```python
from build123d import *

# Parameters (mm, degrees)
F0_W     = 17.78
F0_H     = 12.7
F0_R     = 1.27
F1_DEPTH = 2.54
F2_W     = 2.54
F2_H     = 12.7
F3_DEPTH = 15.24
F4_R     = 1.27
F5_DEPTH = 25.4
F6_SIZE  = 1.27


with BuildPart() as f1:
    # F0 (on Top) → F1 (new body)
    with BuildSketch(Plane.XY):
        with Locations((-26.076857, 25.594209)):
            Rectangle(F0_W, F0_H)
        with Locations((-28.616857, 25.594209)):
            Circle(F0_R, mode=Mode.SUBTRACT)
        with Locations((-20.996857, 25.594209)):
            Circle(F0_R, mode=Mode.SUBTRACT)
    extrude(amount=F1_DEPTH)

    # F2 (on face) → F3 (join)
    with BuildSketch(Plane.XY.offset(2.54)):
        with Locations((-33.696857, 25.594209)):
            Rectangle(F2_W, F2_H)
    extrude(amount=F3_DEPTH)

    # F4 (on face) → F5 (cut)
    with BuildSketch(Plane(origin=(-34.966857, 0, 0), x_dir=(0, -1, 0), z_dir=(-1, 0, 0))):
        with Locations((-25.594209, 13.97)):
            Circle(F4_R)
        with Locations((-25.594209, 6.35)):
            Circle(F4_R)
    extrude(amount=-F5_DEPTH, mode=Mode.SUBTRACT)

    # F6
    f6_edges = [f1.edges().sort_by_distance(p)[0] for p in [
        (-33.696857, 19.244209, 17.78),
        (-33.696857, 31.944209, 17.78),
        (-17.186857, 19.244209, 1.27),
        (-17.186857, 31.944209, 1.27),
    ]]
    chamfer(f6_edges, length=F6_SIZE)


solid = f1.part
```
Work out the finished part from the listing and answer in its coordinate system (mm). A direction names the side the tool comes from. Give positions to 0.01 mm unless a question says otherwise; leave off trailing zeros. Loops run counter-clockwise (first coordinate to the right, second up) from the corner with the lowest first, then second, coordinate; pieces in that order, holes last. Notation, with made-up numbers: M -39.75,-19 L -10.75,-19 A14 cw -10.75,-8 Z; hole C 41.25,72 d11. An arc over 180 degrees is marked long. One line per item, written item: value. Start each with the question number.
1. Find the intervals of material crossed by probe 1 along Z at (x, y) = (-24.5, 24.25); probe 2 along X at (y, z) = (25.5, 3), in increasing order.
2. Find section B-B (y = 27.5). Give the vertices of the cut face in (x, z), and give its area (3 significant figures).
3. Find section D-D (x = -31.25). Give the vertices of the cut face in (y, z), and give its area (3 significant figures).
4. Each of these flat-tipped pins is pushed along its axis until it touches: P1, Ø2, axis at x = -28.62, y = 25.59, coming from the +Z side; P2, Ø5, axis at y = 29, z = 16, coming from the +X side. Where does it stop, or does it pass through?
5. Find section C-C (z = 10.5). Give the vertices of the cut face in (x, y), and give its area (3 significant figures).
6. Find section A-A (z = 13.97). Give the vertices of the cut face in (x, y), and give its area (3 significant figures).
7. Determine the mould class of faces 1 (the face through (-26, 26, 0)), 2 (the face through (-33.715, 24.421, 13.484)), 3 (the face through (-17.8, 19.9, 1.3)), 4 (the face through (-33.715, 24.383, 6.731)) for opening direction Y: released by +Y, released by -Y, zero draft, split by the parting line, or undercut.
8. Which of the six approach directions +Z, -Z, +X, -X, +Y, -Y give full straight-line access (tool end or side, diameter ignored) to faces 5 (the face through (-32.427, 26, 10)), 6 (the face through (-22.266, 25.65, 1.252))?
Reported:
1. probe 1: z = 0 to 2.54
1. probe 2: x = -34.97 to -32.43
2. outline: M -34.97,0 L -17.19,0 L -17.19,2.54 L -32.43,2.54 L -32.43,17.78 L -34.97,17.78 Z
2. area: 83.9 mm²
3. outline: M 19.24,0 L 31.94,0 L 31.94,2.54 L 19.24,2.54 Z
3. area: 32.3 mm²
4. P1: passes through
4. P2: stops at x = -32.43
5. outline: M -34.97,19.24 L -32.43,19.24 L -32.43,31.94 L -34.97,31.94 Z
5. area: 32.3 mm²
6. outline: M -34.97,19.24 L -32.43,19.24 L -32.43,24.32 L -34.97,24.32 Z; M -34.97,26.86 L -32.43,26.86 L -32.43,31.94 L -34.97,31.94 Z
6. area: 25.8 mm²
7. face 1: zero draft
7. face 2: undercut
7. face 3: released by -Y
7. face 4: undercut
8. face 5: +Z, +X, +Y, -Y
8. face 6: +Z, -Z
